The model under review builds one solid part; all positions refer to its coordinate system, in mm. Round coordinates to 2 decimals unless told otherwise and drop trailing zeros. Order: outer loops, then holes, each group sorted by start corner. A loop starts at its lowest first (then second) coordinate and runs counter-clockwise, first axis right, second up. Notation, with made-up numbers: M 50,17.5 L 60,17.5 A27 cw 60,55.5 Z; hole C -11,7 d6. An arc over 180 degrees is marked long. Answer as a JSON object with one key per item and string values. Group by question number.
1) To check wall thickness, follow line 1 (X direction, y = 0.6, z = -14); line 2 (X direction, y = 1.4, z = -47.5); line 3 (X direction, y = 0.5, z = -23.5). State the ranges of each line that lie inside material, in increasing order.
2) Consider section B-B, the plane z = -38. Write out the cut boundary in (x, y), then the cut area to 3 significant figures.
3) Consider section A-A, the plane z = -7. Write out the cut boundary in (x, y).
4) Insertion check: pin 1 Ø0.8 at (x, y) = (38.5, 1) entering from +Z. The pin has a flat end and moves straight along its axis. Give the tip position at first contact, or say it passes through.
5) Consider section C-C, the plane z = -29. Write out the cut boundary in (x, y).
```python
from build123d import *

# Parameters (mm, degrees)
SKETCH1_W               = 234
SKETCH1_H               = 64
BOSS_EXTRUDE1_DEPTH     = 1.5
CUT_EXTRUDE1_DEPTH      = 243.598948885
CUT_EXTRUDE1_DEPTH_BACK = 243.598948885
SKETCH2_W               = 1.5
SKETCH2_H               = 32.5
SKETCH2_H_2             = 1.915
SKETCH2_W_2             = 15
SKETCH2_H_3             = 30


with BuildPart() as part:
    # Sketch1 → Boss-Extrude1 (new body)
    with BuildSketch(Plane(origin=(0, 0, 0), x_dir=(1, 0, 0), z_dir=(0, 1, 0))):
        with Locations((117, 32)):
            Rectangle(SKETCH1_W, SKETCH1_H)
    extrude(amount=BOSS_EXTRUDE1_DEPTH)

    # Sketch2 → Cut-Extrude1 (cut, two sides: drawn at the far end of the back side and taken through both)
    with BuildSketch(Plane(origin=(0, 1.5, 0), x_dir=(1, 0, 0), z_dir=(0, 1, 0)).offset(-CUT_EXTRUDE1_DEPTH_BACK)):
        with Locations((38.333333333, 16.25)):
            Rectangle(SKETCH2_W, SKETCH2_H)
        with Locations((77.666666667, 47.75)):
            Rectangle(SKETCH2_W, SKETCH2_H)
        with Locations((117, 16.25)):
            Rectangle(SKETCH2_W, SKETCH2_H)
        with Locations((195.666666667, 16.25)):
            Rectangle(SKETCH2_W, SKETCH2_H)
        with Locations((156.333333333, 47.75)):
            Rectangle(SKETCH2_W, SKETCH2_H)
        with Locations((0.75, 0.9575)):
            Rectangle(SKETCH2_W, SKETCH2_H_2)
        with Locations((0.75, 63.0425)):
            Rectangle(SKETCH2_W, SKETCH2_H_2)
        with Locations((233.25, 63.0425)):
            Rectangle(SKETCH2_W, SKETCH2_H_2)
        with Locations((233.25, 0.9575)):
            Rectangle(SKETCH2_W, SKETCH2_H_2)
        with Locations((7.5, 32)):
            Rectangle(SKETCH2_W_2, SKETCH2_H_3)
    extrude(amount=CUT_EXTRUDE1_DEPTH + CUT_EXTRUDE1_DEPTH_BACK, mode=Mode.SUBTRACT)


solid = part.part
```
Results list:
{
 "1": {"line 1": "0 to 37.58, 39.08 to 116.25, 117.75 to 194.92, 196.42 to 234", "line 2": "0 to 76.92, 78.42 to 155.58, 157.08 to 234", "line 3": "15 to 37.58, 39.08 to 116.25, 117.75 to 194.92, 196.42 to 234"},
 "2": {"outline": "M 15,0 L 76.92,0 L 76.92,1.5 L 15,1.5 Z; M 78.42,0 L 155.58,0 L 155.58,1.5 L 78.42,1.5 Z; M 157.08,0 L 234,0 L 234,1.5 L 157.08,1.5 Z", "area": "324 mm^2"},
 "3": {"outline": "M 0,0 L 37.58,0 L 37.58,1.5 L 0,1.5 Z; M 39.08,0 L 116.25,0 L 116.25,1.5 L 39.08,1.5 Z; M 117.75,0 L 194.92,0 L 194.92,1.5 L 117.75,1.5 Z; M 196.42,0 L 234,0 L 234,1.5 L 196.42,1.5 Z"},
 "4": {"pin 1": "z = -32.5"},
 "5": {"outline": "M 15,0 L 37.58,0 L 37.58,1.5 L 15,1.5 Z; M 39.08,0 L 116.25,0 L 116.25,1.5 L 39.08,1.5 Z; M 117.75,0 L 194.92,0 L 194.92,1.5 L 117.75,1.5 Z; M 196.42,0 L 234,0 L 234,1.5 L 196.42,1.5 Z"}
}
